For this review, take the finished solid that the model builds, in its own axes (mm). Face numbers are marked on the shaded views. A direction names the side the tool comes from. Coordinates: 2 decimals unless noted, no trailing zeros. Loops run counter-clockwise (first coordinate to the right, second up) from the corner with the lowest first, then second, coordinate; pieces in that order, holes last. Notation, with made-up numbers: (40.25, 39.25) -> (63.25, 39.25) arc R7 ccw to (63.25, 45.25) -> close; hole circle Ø7 at (-11.75, 51). An arc over 180 degrees is marked (long way). Use a Markdown table: item, result.
from build123d import *
from build123d.topology import SkipClean

# Parameters (mm, degrees)
CURVED_HOLDER_MAIN_BODY_SKETCH_R = 3.5
CURVED_HOLDER_MAIN_BODY_DEPTH    = 5
FILL_REMOVE_DEPTH                = 8.03562364
FILL_REMOVE_DEPTH_BACK           = 8.03562364
PIN_BODY_REACH                   = 7.036
PIN_BODY_END_RADIUS              = 15
PIN_BODY_SKETCH_R                = 1.5
PIN_BODY_DIRECTION_2_DEPTH       = 7.5


with BuildPart() as part:
    # Curved Holder Main Body Sketch → Curved Holder Main Body (new body)
    with BuildSketch(Plane.XY):
        Circle(CURVED_HOLDER_MAIN_BODY_SKETCH_R)
    extrude(amount=CURVED_HOLDER_MAIN_BODY_DEPTH)

    # Fill Remove Sketch → Fill Remove (cut, two sides: drawn at the far end of the back side and taken through both)
    with BuildSketch(Plane(origin=(0, 0, 0), x_dir=(1, 0, 0), z_dir=(0, 1, 0)).offset(-FILL_REMOVE_DEPTH_BACK)):
        with BuildLine():
            Line((3.5, -5), (3.5, -0.928752721))
            ThreePointArc((3.5, -0.928752721), (0, -0.5), (-3.5, -0.928752721))
            Line((-3.5, -0.928752721), (-3.5, -5))
            Line((-3.5, -5), (3.5, -5))
        make_face()
        with BuildLine():
            Line((-3.5, 0), (-3.5, -0.414047854))
            ThreePointArc((-3.5, -0.414047854), (0, 0), (3.5, -0.414047854))
            Line((3.5, -0.414047854), (3.5, 0))
            Line((3.5, 0), (3.5, 0.978197193))
            Line((3.5, 0.978197193), (-3.5, 0.978197193))
            Line((-3.5, 0.978197193), (-3.5, 0))
        make_face()
    extrude(amount=FILL_REMOVE_DEPTH + FILL_REMOVE_DEPTH_BACK, mode=Mode.SUBTRACT)

    # Pin Body: up to this cylinder (the profile starts outside it)
    with SkipClean():  # the faces are left unmerged after this step: merging them gives an invalid solid
        pin_body_end = Plane(origin=(0, 0, 15), z_dir=(0, 1, 0)) * Cylinder(PIN_BODY_END_RADIUS, 45.072, mode=Mode.PRIVATE)
        # Pin Body Sketch → Pin Body (add, up to the surface)
        with BuildSketch(Plane.XY, mode=Mode.PRIVATE) as pin_body_sk1:
            Circle(PIN_BODY_SKETCH_R)
        pin_body_tool1 = extrude(pin_body_sk1.sketch, amount=PIN_BODY_REACH, mode=Mode.PRIVATE) - pin_body_end
        add(pin_body_tool1.solids().sort_by_distance((0, 0, 0))[0])
        add(pin_body_tool1.solids().sort_by_distance((0, 0, 0))[1])

    # Pin Body Sketch → Pin Body direction 2 (add)
    with BuildSketch(Plane.XY):
        Circle(PIN_BODY_SKETCH_R)
    extrude(amount=-PIN_BODY_DIRECTION_2_DEPTH)


solid = part.part
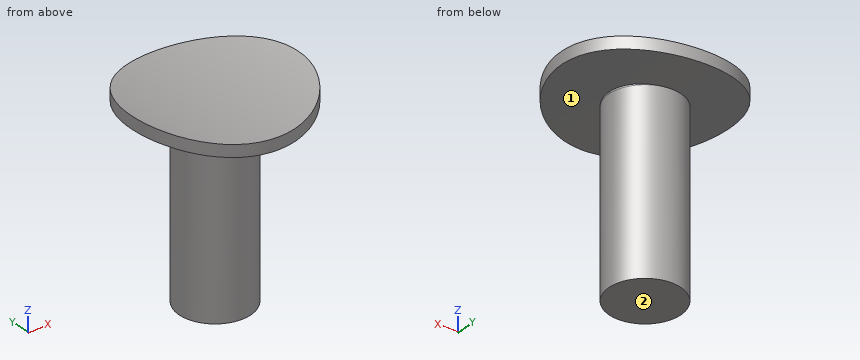
(1) For pin 1 Ø1.5 at (x, y) = (1, 2.5) entering from +Z; pin 2 Ø1 at (y, z) = (1.5, -1.5) entering from +X; pin 3 Ø1.5 at (x, z) = (1, -4.5) entering from +Y, all flat-tipped, find the tip position at first contact; note any pin that passes through.
Found:
| item | result |
|---|---|
| pin 1 | stops at z = 0.61 |
| pin 2 | stops at x = 1.12 |
| pin 3 | stops at y = 1.48 |
(2) For the marked faces 1 and 2, list the 3-axis set-ups (+Z, -Z, +X, -X, +Y, -Y) from which the entire face can be reached by the end or side of a thin tool; tool diameter is ignored.
Found:
| item | result |
|---|---|
| face 1 | -Z |
| face 2 | -Z, +X, -X, +Y, -Y |
(3) Take a section at A-A on y = -1. Write out the cut boundary in (x, z), plus the area to 3 significant figures.
Found:
| item | result |
|---|---|
| outline | (-3.35, 0.38) arc R15 ccw to (-1.12, 0.04) -> (-1.12, -7.5) -> (1.12, -7.5) -> (1.12, 0.04) arc R15 ccw to (3.35, 0.38) -> (3.35, 0.89) arc R14.5 cw to (-3.35, 0.89) -> close |
| area | 20.2 mm^2 |
(4) Take a section at B-B on x = 1.25. Write out the cut boundary in (y, z), plus the area to 3 significant figures.
Found:
| item | result |
|---|---|
| outline | (-3.27, 0.05) -> (-0.83, 0.05) -> (-0.83, -7.5) -> (0.83, -7.5) -> (0.83, 0.05) -> (3.27, 0.05) -> (3.27, 0.55) -> (-3.27, 0.55) -> close |
| area | 15.8 mm^2 |
(5) For line 1 along Z through (x, y) = (0.25, -2); line 2 along Y through (x, z) = (0, -5.5); line 3 along X through (y, z) = (-0.75, -2.75), list the stretches that pass through material, from the lowest coordinate up.
Found:
| item | result |
|---|---|
| line 1 | z = 0 to 0.5 |
| line 2 | y = -1.5 to 1.5 |
| line 3 | x = -1.3 to 1.3 |
(6) Take a section at C-C on z = -6.5. Write out the cut boundary in (x, y), plus the area to 3 significant figures.
Found:
| item | result |
|---|---|
| outline | circle Ø3 at (0, 0) |
| area | 7.07 mm^2 |
(7) Take a section at D-D on x = -3. Write out the cut boundary in (y, z).
Found:
| item | result |
|---|---|
| outline | (-1.8, 0.3) -> (1.8, 0.3) -> (1.8, 0.81) -> (-1.8, 0.81) -> close |
